Check sheet for the modelled part. Datum: model origin and axes. Units: mm. A direction names the side the tool comes from. Coordinates: 2 decimals unless noted, no trailing zeros. Write each loop counter-clockwise with the first axis right and the second up, starting at its lowest first coordinate (ties: lowest second). Pieces come first, ordered by that corner, then holes. Notation, with made-up numbers: M 43.25,8 L 72.25,8 A27 ccw 72.25,44 Z; hole C 46,8 d7. An arc over 180 degrees is marked long. Answer as CSV lines item,"result". Start each with the question number.
Q1. Sectioned sample at C-C, the plane z = 2.5. Record the cut outline in (x, y).
Q2. Thickness scan on line 1 along Y through (x, z) = (-57.5, 5.75); line 2 along X through (y, z) = (-0.75, 2.5); line 3 along X through (y, z) = (-4.75, 6.5). Record the ranges inside material, lowest first. Write a range as from..to.
Q3. Mould release check, pull along Y, two halves, no side actions. Record for faces 3 (the flat face through (0, 9, 10)), 4 (the cylindrical face through (84, 0, 5)), 5 (the flat face through (-1, 8.5, 5)), 6 (the cylindrical face through (-87, 0, 5)): pulls with the +Y half, pulls with the -Y half, needs draft (parallel to the pull), parting line crosses it, or undercut.
Q4. Sectioned sample at A-A, the plane x = -73. Record the cut outline in (y, z), then the cut area to 3 significant figures.
Q5. Sectioned sample at B-B, the plane y = 0. Record the cut outline in (x, z), then the cut area to 3 significant figures.
Q6. Access from +Z, -Z, +X, -X, +Y, -Y to the whole of each face (thin tool, end or side, straight path). Record for faces 1 (the cylindrical face through (87, 0, 5)), 2 (the flat face through (-1, -8.5, 5)).
Q7. Depth check by flat-ended pin: pin 1 Ø4 at (y, z) = (-9, 5) entering from -X. Enter the tip coordinate at first touch or a pass-through.
Autodesk Inventor part; units mm, degrees
ref_plane "YZ Plane" through (0, 0, 0) normal (1, 0, 0) x (0, 1, 0)
ref_plane "XZ Plane" through (0, 0, 0) normal (0, 1, 0) x (-1, 0, 0)
ref_plane "XY Plane" through (0, 0, 0) normal (0, 0, 1) x (1, 0, 0)
sketch "Sketch1" plane through (0, 0, 0) normal (0, 0, 1) x (1, 0, 0)
  line L0 (-75.5, 11.5) -> (75.5, 11.5)
  line L1 (75.5, -11.5) -> (-75.5, -11.5)
  arc A0 (-75.5, 11.5) -> (-75.5, -11.5) centre (-75.5, 0) ccw
  arc A1 (75.5, -11.5) -> (75.5, 11.5) centre (75.5, 0) ccw
  line L2 (-75.5, 8.5) -> (75.5, 8.5)
  line L3 (-75.5, -8.5) -> (75.5, -8.5)
  arc A2 (-75.5, 8.5) -> (-75.5, -8.5) centre (-75.5, 0) ccw
  arc A3 (75.5, -8.5) -> (75.5, 8.5) centre (75.5, 0) ccw
  point P0 (0, 0)
  point P1 (0, 8.5)
  point P2 (0, 11.5)
  dimension "d0" = 151
  dimension "d1" = 23
  dimension "d2" = 3
  dimension "d3" = 3
  dimension "d4" = 11.5
  dimension "d5" = 8.5
  dimension "d7" = 8.5
  dimension "d8" = 151
  dimension "d9" = 151
extrude "Extrusion1" add sketch "Sketch1" along normal blind 10
properties part number "faja" material "Rubber, Silicone"
Output:
1,outline,"M -75.5,-11.5 L 75.5,-11.5 A11.5 ccw 75.5,11.5 L -75.5,11.5 A11.5 ccw Z; hole M -75.5,-8.5 L 75.5,-8.5 A8.5 ccw 75.5,8.5 L -75.5,8.5 A8.5 ccw Z"
2,line 1,"y = -11.5..-8.5, 8.5..11.5"
2,line 2,"x = -86.98..-83.97, 83.97..86.98"
2,line 3,"x = -85.97..-82.55, 82.55..85.97"
3,face 3,"needs draft"
3,face 4,"undercut"
3,face 5,"undercut"
3,face 6,"parting line crosses it"
4,outline,"M -11.5,0 L -8.5,0 L -8.5,10 L -11.5,10 Z; M 8.5,0 L 11.5,0 L 11.5,10 L 8.5,10 Z"
4,area,"60.0 mm^2"
5,outline,"M -87,0 L -84,0 L -84,10 L -87,10 Z; M 84,0 L 87,0 L 87,10 L 84,10 Z"
5,area,"60.0 mm^2"
6,face 1,"+Z, -Z, +X"
6,face 2,"+Z, -Z"
7,pin 1,"stops at x = -84.62"
